from build123d import *

# Parameters (mm, degrees)
SKETCH1_R           = 25.4
BOSS_EXTRUDE1_DEPTH = 3.81
SKETCH1_3_R         = 25.4
BOSS_EXTRUDE2_DEPTH = 22.225


with BuildPart() as part:
    # Sketch1 → Boss-Extrude1 (new body)
    with BuildSketch(Plane.XY):
        with BuildLine():
            Line((-1.016, 38.989), (1.016, 38.989))
            Line((1.016, 38.989), (2.402726593, 35.179))
            ThreePointArc((2.402726593, 35.179), (4.418420371, 33.561234708), (6.784139518, 34.602176045))
            Line((6.784139518, 34.602176045), (9.10971511, 37.923442191))
            Line((9.10971511, 37.923442191), (11.072476389, 37.397521891))
            Line((11.072476389, 37.397521891), (11.425850857, 33.358433241))
            ThreePointArc((11.425850857, 33.358433241), (12.954153068, 31.274092025), (15.508677732, 31.667270976))
            Line((15.508677732, 31.667270976), (18.61461819, 34.273464468))
            Line((18.61461819, 34.273464468), (20.37438181, 33.257464468))
            Line((20.37438181, 33.257464468), (19.670322268, 29.264544383))
            ThreePointArc((19.670322268, 29.264544383), (20.60708164, 26.855671653), (23.176325188, 26.574293722))
            Line((23.176325188, 26.574293722), (26.850965802, 28.287806781))
            Line((26.850965802, 28.287806781), (28.287806781, 26.850965802))
            Line((28.287806781, 26.850965802), (26.574293722, 23.176325188))
            ThreePointArc((26.574293722, 23.176325188), (26.855671653, 20.60708164), (29.264544383, 19.670322268))
            Line((29.264544383, 19.670322268), (33.257464468, 20.37438181))
            Line((33.257464468, 20.37438181), (34.273464468, 18.61461819))
            Line((34.273464468, 18.61461819), (31.667270976, 15.508677732))
            ThreePointArc((31.667270976, 15.508677732), (31.274092025, 12.954153068), (33.358433241, 11.425850857))
            Line((33.358433241, 11.425850857), (37.397521891, 11.072476389))
            Line((37.397521891, 11.072476389), (37.923442191, 9.10971511))
            Line((37.923442191, 9.10971511), (34.602176045, 6.784139518))
            ThreePointArc((34.602176045, 6.784139518), (33.561234708, 4.418420371), (35.179, 2.402726593))
            Line((35.179, 2.402726593), (38.989, 1.016))
            Line((38.989, 1.016), (38.989, -1.016))
            Line((38.989, -1.016), (35.179, -2.402726593))
            ThreePointArc((35.179, -2.402726593), (33.561234708, -4.418420371), (34.602176045, -6.784139518))
            Line((34.602176045, -6.784139518), (37.923442191, -9.10971511))
            Line((37.923442191, -9.10971511), (37.397521891, -11.072476389))
            Line((37.397521891, -11.072476389), (33.358433241, -11.425850857))
            ThreePointArc((33.358433241, -11.425850857), (31.274092025, -12.954153068), (31.667270976, -15.508677732))
            Line((31.667270976, -15.508677732), (34.273464468, -18.61461819))
            Line((34.273464468, -18.61461819), (33.257464468, -20.37438181))
            Line((33.257464468, -20.37438181), (29.264544383, -19.670322268))
            ThreePointArc((29.264544383, -19.670322268), (26.855671653, -20.60708164), (26.574293722, -23.176325188))
            Line((26.574293722, -23.176325188), (28.287806781, -26.850965802))
            Line((28.287806781, -26.850965802), (26.850965802, -28.287806781))
            Line((26.850965802, -28.287806781), (23.176325188, -26.574293722))
            ThreePointArc((23.176325188, -26.574293722), (20.60708164, -26.855671653), (19.670322268, -29.264544383))
            Line((19.670322268, -29.264544383), (20.37438181, -33.257464468))
            Line((20.37438181, -33.257464468), (18.61461819, -34.273464468))
            Line((18.61461819, -34.273464468), (15.508677732, -31.667270976))
            ThreePointArc((15.508677732, -31.667270976), (12.954153068, -31.274092025), (11.425850857, -33.358433241))
            Line((11.425850857, -33.358433241), (11.072476389, -37.397521891))
            Line((11.072476389, -37.397521891), (9.10971511, -37.923442191))
            Line((9.10971511, -37.923442191), (6.784139518, -34.602176045))
            ThreePointArc((6.784139518, -34.602176045), (4.418420371, -33.561234708), (2.402726593, -35.179))
            Line((2.402726593, -35.179), (1.016, -38.989))
            Line((1.016, -38.989), (-1.016, -38.989))
            Line((-1.016, -38.989), (-2.402726593, -35.179))
            ThreePointArc((-2.402726593, -35.179), (-4.418420371, -33.561234708), (-6.784139518, -34.602176045))
            Line((-6.784139518, -34.602176045), (-9.10971511, -37.923442191))
            Line((-9.10971511, -37.923442191), (-11.072476389, -37.397521891))
            Line((-11.072476389, -37.397521891), (-11.425850857, -33.358433241))
            ThreePointArc((-11.425850857, -33.358433241), (-12.954153068, -31.274092025), (-15.508677732, -31.667270976))
            Line((-15.508677732, -31.667270976), (-18.61461819, -34.273464468))
            Line((-18.61461819, -34.273464468), (-20.37438181, -33.257464468))
            Line((-20.37438181, -33.257464468), (-19.670322268, -29.264544383))
            ThreePointArc((-19.670322268, -29.264544383), (-20.60708164, -26.855671653), (-23.176325188, -26.574293722))
            Line((-23.176325188, -26.574293722), (-26.850965802, -28.287806781))
            Line((-26.850965802, -28.287806781), (-28.287806781, -26.850965802))
            Line((-28.287806781, -26.850965802), (-26.574293722, -23.176325188))
            ThreePointArc((-26.574293722, -23.176325188), (-26.855671653, -20.60708164), (-29.264544383, -19.670322268))
            Line((-29.264544383, -19.670322268), (-33.257464468, -20.37438181))
            Line((-33.257464468, -20.37438181), (-34.273464468, -18.61461819))
            Line((-34.273464468, -18.61461819), (-31.667270976, -15.508677732))
            ThreePointArc((-31.667270976, -15.508677732), (-31.274092025, -12.954153068), (-33.358433241, -11.425850857))
            Line((-33.358433241, -11.425850857), (-37.397521891, -11.072476389))
            Line((-37.397521891, -11.072476389), (-37.923442191, -9.10971511))
            Line((-37.923442191, -9.10971511), (-34.602176045, -6.784139518))
            ThreePointArc((-34.602176045, -6.784139518), (-33.561234708, -4.418420371), (-35.179, -2.402726593))
            Line((-35.179, -2.402726593), (-38.989, -1.016))
            Line((-38.989, -1.016), (-38.989, 1.016))
            Line((-38.989, 1.016), (-35.179, 2.402726593))
            ThreePointArc((-35.179, 2.402726593), (-33.561234708, 4.418420371), (-34.602176045, 6.784139518))
            Line((-34.602176045, 6.784139518), (-37.923442191, 9.10971511))
            Line((-37.923442191, 9.10971511), (-37.397521891, 11.072476389))
            Line((-37.397521891, 11.072476389), (-33.358433241, 11.425850857))
            ThreePointArc((-33.358433241, 11.425850857), (-31.274092025, 12.954153068), (-31.667270976, 15.508677732))
            Line((-31.667270976, 15.508677732), (-34.273464468, 18.61461819))
            Line((-34.273464468, 18.61461819), (-33.257464468, 20.37438181))
            Line((-33.257464468, 20.37438181), (-29.264544383, 19.670322268))
            ThreePointArc((-29.264544383, 19.670322268), (-26.855671653, 20.60708164), (-26.574293722, 23.176325188))
            Line((-26.574293722, 23.176325188), (-28.287806781, 26.850965802))
            Line((-28.287806781, 26.850965802), (-26.850965802, 28.287806781))
            Line((-26.850965802, 28.287806781), (-23.176325188, 26.574293722))
            ThreePointArc((-23.176325188, 26.574293722), (-20.60708164, 26.855671653), (-19.670322267, 29.264544383))
            Line((-19.670322267, 29.264544383), (-20.37438181, 33.257464468))
            Line((-20.37438181, 33.257464468), (-18.61461819, 34.273464468))
            Line((-18.61461819, 34.273464468), (-15.508677732, 31.667270976))
            ThreePointArc((-15.508677732, 31.667270976), (-12.954153068, 31.274092025), (-11.425850857, 33.358433241))
            Line((-11.425850857, 33.358433241), (-11.072476389, 37.397521891))
            Line((-11.072476389, 37.397521891), (-9.10971511, 37.923442191))
            Line((-9.10971511, 37.923442191), (-6.784139518, 34.602176045))
            ThreePointArc((-6.784139518, 34.602176045), (-4.418420371, 33.561234708), (-2.402726593, 35.179))
            Line((-2.402726593, 35.179), (-1.016, 38.989))
        make_face()
        with Locations(Location((0, 0, 0), (0, 0, 180))):
            Circle(SKETCH1_R, mode=Mode.SUBTRACT)
    extrude(amount=BOSS_EXTRUDE1_DEPTH)

    # Sketch1_3 → Boss-Extrude2 (add)
    with BuildSketch(Plane.XY):
        Circle(SKETCH1_3_R)
        with BuildLine():
            ThreePointArc((-3.175, 12.296722124), (0, -12.7), (3.175, 12.296722124))
            Line((3.175, 12.296722124), (3.175, 15.875))
            Line((3.175, 15.875), (-3.175, 15.875))
            Line((-3.175, 15.875), (-3.175, 12.296722124))
        make_face(mode=Mode.SUBTRACT)
    extrude(amount=BOSS_EXTRUDE2_DEPTH)


solid = part.part
Design review of the part built by this model. Coordinates are the model's own, in mm. A direction names the side the tool comes from. Round coordinates to 2 decimals unless told otherwise and drop trailing zeros. Loops run counter-clockwise (first coordinate to the right, second up) from the corner with the lowest first, then second, coordinate; pieces in that order, holes last. Notation, with made-up numbers: (-13.5, 37) -> (35.5, 37) arc R17 cw to (35.5, 49) -> close; hole circle Ø7 at (0.5, 46). An arc over 180 degrees is marked (long way). Use one line per item in the form item = value. Start each with the question number.
Q1. We need section A-A on y = 0. Give the boundary of the cut face in (x, z) (3 decimals), then the cut area to 3 significant figures.
Q2. Wall thickness on line 1 along Y through (x, z) = (0, 13) (3 decimals); line 2 along Y through (x, z) = (32, 2.5); line 3 along Y through (x, z) = (32.5, 1.25): over which ranges is each line inside the solid? List them lowest first. Write a range as [from, to].
Q3. Draft analysis for pull direction X (two halves, no side actions). For faces 1 (the face through (31.26, 12.99, 1.88)), 2 (the face through (-35.35, -11.25, 1.88)), 3 (the face through (31.233, 20.017, 1.878)), state which applies: +X half, -X half, draft (parallel to the pull), parting line (faces both ways), or undercut.
Q4. We need section C-C on x = 0. Give the boundary of the cut face in (y, z) (3 decimals).
Q5. We need section B-B on z = 7. Give the boundary of the cut face in (x, y) (3 decimals).
Q6. Machinability: for faces 4 (the face through (20.027, 31.289, 1.878)), 5 (the face through (1.72, -37.06, 1.88)), 6 (the face through (-19.507, 33.758, 1.878)), 7 (the face through (-20.017, 31.233, 1.878)), 8 (the face through (24.99, 27.42, 1.88)), which of the approach directions +Z, -Z, +X, -X, +Y, -Y give a long, thin tool a straight path to every point of the face, cutting with its end or side? Answer none if there is none.
Q7. For pin 1 Ø1.5 at (y, z) = (13.5, 12.5) entering from +X; pin 2 Ø8 at (x, y) = (-13.5, -24) entering from -Z; pin 3 Ø1.8 at (y, z) = (14.5, 14.5) entering from -X; pin 4 Ø8 at (y, z) = (27, 15) entering from -X, all flat-tipped, find the tip position at first contact; note any pin that passes through.
Calculated:
q1.outline = (-38.989, 0) -> (-12.7, 0) -> (-12.7, 22.225) -> (-25.4, 22.225) -> (-25.4, 3.81) -> (-38.989, 3.81) -> close; (12.7, 0) -> (38.989, 0) -> (38.989, 3.81) -> (25.4, 3.81) -> (25.4, 22.225) -> (12.7, 22.225) -> close
q1.area = 668 mm²
q2.line_1 = [-25.4, -12.7], [15.875, 25.4]
q2.line_2 = [-20.15, -15.91], [-11.98, 11.98], [15.91, 20.15]
q2.line_3 = [-20.24, -16.5], [-11.66, 11.66], [16.5, 20.24]
q3.face_1 = +X half
q3.face_2 = -X half
q3.face_3 = undercut
q4.outline = (-38.989, 0) -> (-12.7, 0) -> (-12.7, 22.225) -> (-25.4, 22.225) -> (-25.4, 3.81) -> (-38.989, 3.81) -> close; (15.875, 0) -> (38.989, 0) -> (38.989, 3.81) -> (25.4, 3.81) -> (25.4, 22.225) -> (15.875, 22.225) -> close
q5.outline = circle Ø50.8 at (0, 0); hole (-3.175, 12.297) arc R12.7 ccw (long way) to (3.175, 12.297) -> (3.175, 15.875) -> (-3.175, 15.875) -> close
q6.face_4 = +Z, -Z, +X
q6.face_5 = +Z, -Z, -Y
q6.face_6 = +Z, -Z, -X, +Y
q6.face_7 = +Z, -Z, -X
q6.face_8 = +Z, -Z, +Y
q7.pin_1 = 21.97
q7.pin_2 = 0
q7.pin_3 = -21.45
q7.pin_4 = -10.78
